The model under review builds one solid part; all positions refer to its coordinate system, in mm. A direction names the side the tool comes from. Give positions to 0.01 mm unless a question says otherwise; leave off trailing zeros. Order: outer loops, then holes, each group sorted by start corner. A loop starts at its lowest first (then second) coordinate and runs counter-clockwise, first axis right, second up.
```python
from build123d import *

# Parameters (mm, degrees)
BOSS_EXTRUDE1_DEPTH = 10
SKETCH2_R           = 6.75
SKETCH2_R_2         = 1.65
CUT_EXTRUDE1_DEPTH  = 97.21752699
SKETCH3_W           = 15
SKETCH3_H           = 5
SKETCH4_R           = 10
BOSS_EXTRUDE2_DEPTH = 15
SKETCH5_R           = 8.5
CUT_EXTRUDE2_DEPTH  = 7


with BuildPart() as part:
    # Sketch1 → Boss-Extrude1 (new body)
    with BuildSketch(Plane.XY):
        with BuildLine():
            ThreePointArc((35.510171199, 15.510971646), (-38.75, 0), (35.510171199, -15.510971646))
            Line((35.510171199, -15.510971646), (77.5, -10))
            ThreePointArc((77.5, -10), (87.5, 0), (77.5, 10))
            Line((77.5, 10), (35.510171199, 15.510971646))
        make_face()
    extrude(amount=BOSS_EXTRUDE1_DEPTH)

    # Sketch2 → Cut-Extrude1 (cut, through all)
    with BuildSketch(Plane.XY.offset(10)):
        Circle(SKETCH2_R)
        with Locations((12, 0)):
            Circle(SKETCH2_R_2)
        with Locations((6, -10.392304845)):
            Circle(SKETCH2_R_2)
        with Locations((-6, -10.392304845)):
            Circle(SKETCH2_R_2)
        with Locations((-12, 0)):
            Circle(SKETCH2_R_2)
        with Locations((-6, 10.392304845)):
            Circle(SKETCH2_R_2)
        with Locations((6, 10.392304845)):
            Circle(SKETCH2_R_2)
    extrude(amount=-CUT_EXTRUDE1_DEPTH, mode=Mode.SUBTRACT)

    # Sketch3 → Cut-Revolve1 (revolve, cut)
    with BuildSketch(Plane(origin=(0, 0, 0), x_dir=(1, 0, 0), z_dir=(0, 1, 0))):
        with Locations((7.5, -2.5)):
            Rectangle(SKETCH3_W, SKETCH3_H)
        Polygon((15, -5), (20, 0), (15, 0), align=None)
    revolve(axis=Axis((0, 0, 0), (0, 0, 1)), mode=Mode.SUBTRACT)

    # Sketch4 → Boss-Extrude2 (add)
    with BuildSketch(Plane(origin=(0, 0, 0), x_dir=(-1, 0, 0), z_dir=(0, 0, -1))):
        with Locations((-77.5, 0)):
            Circle(SKETCH4_R)
    extrude(amount=-BOSS_EXTRUDE2_DEPTH)

    # Sketch5 → Cut-Extrude2 (cut)
    with BuildSketch(Plane.XY.offset(15)):
        with Locations((77.5, 0)):
            Circle(SKETCH5_R)
    extrude(amount=-CUT_EXTRUDE2_DEPTH, mode=Mode.SUBTRACT)


solid = part.part
```
Item 1: Clearance check with flat-ended pins moving along their axes: pin 1 Ø1 at (y, z) = (-6.5, 13) entering from -X; pin 2 Ø5.5 at (x, y) = (-6, -10.39) entering from -Z; pin 3 Ø1.5 at (y, z) = (-23, 4) entering from +X; pin 4 Ø19.5 at (x, y) = (77.5, 0) entering from -Z. State where each tip first meets the part, or that it passes through.
Values found:
pin 1: stops at x = 69.5
pin 2: stops at z = 5
pin 3: stops at x = 31.73
pin 4: stops at z = 0
Item 2: Take a section at B-B (z = 3.5). Give the boundary of the cut face in (x, y).
Values found:
outline: (35.51, -15.51) - (77.5, -10) arc R10 ccw to (77.5, 10) - (35.51, 15.51) arc R38.75 ccw (long way) to start; hole circle Ø33 at (0, 0)
Item 3: For line 1 (Z direction, x = 35, y = -6); line 2 (Y direction, x = 8, z = 4); line 3 (X direction, y = -2, z = 4.5), list the stretches that pass through material, from the lowest coordinate up.
Values found:
line 1: z = 0 to 10
line 2: y = -37.92 to -13.86, 13.86 to 37.92
line 3: x = -38.7 to -15.37, 15.37 to 87.3
Item 4: Draft analysis for pull direction Y (two halves, no side actions). For faces 1 (the cylindrical face through (69, 0, 12)), 2 (the flat face through (82, -7.4, 15)), 3 (the cylindrical face through (-38.72, 1.48, 4.93)), state which applies: released by +Y, released by -Y, zero draft, split by the parting line, or undercut.
Values found:
face 1: undercut
face 2: zero draft
face 3: split by the parting line
Item 5: Take a section at A-A (x = 0). Give the boundary of the cut face in (y, z).
Values found:
outline: (-38.75, 0) - (-20, 0) - (-15, 5) - (-6.75, 5) - (-6.75, 10) - (-38.75, 10) - close; (6.75, 5) - (15, 5) - (20, 0) - (38.75, 0) - (38.75, 10) - (6.75, 10) - close
Item 6: For faces 4 (the flat face through (77, 0, 8)), 5 (the cylindrical face through (4.691, -11.396, 7.535)), 6 (the flat face through (-3.1, -6.5, 5)), list the 3-axis set-ups (+Z, -Z, +X, -X, +Y, -Y) from which the entire face can be reached by the end or side of a thin tool; tool diameter is ignored.
Values found:
face 4: +Z
face 5: +Z, -Z
face 6: -Z
Item 7: Take a section at D-D (y = -21.5). Give the boundary of the cut face in (x, z), and give its area (3 significant figures).
Values found:
outline: (-32.24, 0) - (32.24, 0) - (32.24, 10) - (-32.24, 10) - close
area: 645 mm2
Item 8: Take a section at C-C (x = 70.5). Give the boundary of the cut face in (y, z).
Values found:
outline: (-10.92, 0) - (10.92, 0) - (10.92, 10) - (7.14, 10) - (7.14, 15) - (4.82, 15) - (4.82, 8) - (-4.82, 8) - (-4.82, 15) - (-7.14, 15) - (-7.14, 10) - (-10.92, 10) - close
